from build123d import *

# Parameters (mm, degrees)
SKETCH1_W               = 95.2
SKETCH1_H               = 59.2
BOSS_EXTRUDE1_DEPTH     = 2
SKETCH2_R               = 6.5
CUT_EXTRUDE2_DEPTH      = 1
CUT_EXTRUDE2_DEPTH_BACK = 3
FILLET1_R               = 17.6


with BuildPart() as part:
    # Sketch1 → Boss-Extrude1 (new body)
    with BuildSketch(Plane(origin=(0, 0, 0), x_dir=(0, 1, 0), z_dir=(0, 0, 1))):
        with Locations((0, 29.6)):
            Rectangle(SKETCH1_W, SKETCH1_H)
    extrude(amount=BOSS_EXTRUDE1_DEPTH)

    # Sketch2 → Cut-Extrude2 (cut, two sides)
    with BuildSketch(Plane.XY.offset(2)) as cut_extrude2_sk:
        with Locations((-29.6, 0)):
            Circle(SKETCH2_R)
        with Locations((-46.6, 0)):
            Circle(SKETCH2_R)
        with Locations((-12.6, 0)):
            Circle(SKETCH2_R)
        with Locations((-12.6, -17)):
            Circle(SKETCH2_R)
        with Locations((-46.6, -17)):
            Circle(SKETCH2_R)
        with Locations((-29.6, -17)):
            Circle(SKETCH2_R)
        with Locations((-12.6, -34)):
            Circle(SKETCH2_R)
        with Locations((-46.6, -34)):
            Circle(SKETCH2_R)
        with Locations((-29.6, -34)):
            Circle(SKETCH2_R)
        with Locations((-46.6, 17)):
            Circle(SKETCH2_R)
        with Locations((-29.6, 17)):
            Circle(SKETCH2_R)
        with Locations((-12.6, 17)):
            Circle(SKETCH2_R)
        with Locations((-46.6, 34)):
            Circle(SKETCH2_R)
        with Locations((-29.6, 34)):
            Circle(SKETCH2_R)
        with Locations((-12.6, 34)):
            Circle(SKETCH2_R)
    extrude(amount=CUT_EXTRUDE2_DEPTH, mode=Mode.SUBTRACT)
    extrude(cut_extrude2_sk.sketch, amount=-CUT_EXTRUDE2_DEPTH_BACK, mode=Mode.SUBTRACT)

    # Fillet1
    fillet1_edges = [part.edges().sort_by_distance(p)[0] for p in [
        (-59.2, -47.6, 1),
        (-59.2, 47.6, 1),
        (0, 47.6, 1),
        (0, -47.6, 1),
    ]]
    fillet(fillet1_edges, radius=FILLET1_R)


solid = part.part
For this review, take the finished solid that the model builds, in its own axes (mm). Coordinates: 2 decimals unless noted, no trailing zeros. Loops run counter-clockwise (first coordinate to the right, second up) from the corner with the lowest first, then second, coordinate; pieces in that order, holes last. Notation, with made-up numbers: (72.25, 88.25) - (81.25, 88.25) arc R34 ccw to (81.25, 118.25) - close; hole circle Ø10 at (-27, 47). An arc over 180 degrees is marked (long way). Use a Markdown table: item, result. Add a question column.
Item 1: We need section D-D (y = -34). Give the boundary of the cut face in (x, z).
Item 2: We need section B-B (z = 1.15). Give the number of separate pieces and of enclosed holes in the cut face, and give its area (3 significant figures).
Item 3: We need section C-C (x = -34). Give the boundary of the cut face in (y, z).
Item 4: Mouldability with a two-part tool opening along X and no side actions: class faces 1 (the face through (-54.18, 42.31, 1.01)), 2 (the face through (-13.446, -27.555, 1.014)), 3 (the face through (-37, -1, 2)) as pulls with the +X half, pulls with the -X half, needs draft (parallel to the pull), parting line crosses it, or undercut.
Item 5: We need section A-A (y = 17). Give the boundary of the cut face in (x, z).
Item 6: Insertion check: pin 1 Ø8 at (x, y) = (-29.6, -17) entering from -Z. The pin has a flat end and moves straight along its axis. Give the tip position at first contact, or say it passes through.
Item 7: For line 1 (Y direction, x = -29.6, z = 0.6); line 2 (Y direction, x = -28, z = 1.45); line 3 (X direction, y = -0.5, z = 1.3), list the stretches that pass through material, from the lowest coordinate up.
Results list:
| question | item | result |
|---|---|---|
| 1 | outline | (-58.74, 0) - (-53.1, 0) - (-53.1, 2) - (-58.74, 2) - close; (-40.1, 0) - (-36.1, 0) - (-36.1, 2) - (-40.1, 2) - close; (-23.1, 0) - (-19.1, 0) - (-19.1, 2) - (-23.1, 2) - close; (-6.1, 0) - (-0.46, 0) - (-0.46, 2) - (-6.1, 2) - close |
| 2 | separate pieces | 1 |
| 2 | enclosed holes | 15 |
| 2 | area | 3,380 mm^2 |
| 3 | outline | (-47.6, 0) - (-38.78, 0) - (-38.78, 2) - (-47.6, 2) - close; (-29.22, 0) - (-21.78, 0) - (-21.78, 2) - (-29.22, 2) - close; (-12.22, 0) - (-4.78, 0) - (-4.78, 2) - (-12.22, 2) - close; (4.78, 0) - (12.22, 0) - (12.22, 2) - (4.78, 2) - close; (21.78, 0) - (29.22, 0) - (29.22, 2) - (21.78, 2) - close; (38.78, 0) - (47.6, 0) - (47.6, 2) - (38.78, 2) - close |
| 4 | face 1 | pulls with the -X half |
| 4 | face 2 | undercut |
| 4 | face 3 | needs draft |
| 5 | outline | (-59.2, 0) - (-53.1, 0) - (-53.1, 2) - (-59.2, 2) - close; (-40.1, 0) - (-36.1, 0) - (-36.1, 2) - (-40.1, 2) - close; (-23.1, 0) - (-19.1, 0) - (-19.1, 2) - (-23.1, 2) - close; (-6.1, 0) - (0, 0) - (0, 2) - (-6.1, 2) - close |
| 6 | pin 1 | passes through |
| 7 | line 1 | y = -47.6 to -40.5, -27.5 to -23.5, -10.5 to -6.5, 6.5 to 10.5, 23.5 to 27.5, 40.5 to 47.6 |
| 7 | line 2 | y = -47.6 to -40.3, -27.7 to -23.3, -10.7 to -6.3, 6.3 to 10.7, 23.3 to 27.7, 40.3 to 47.6 |
| 7 | line 3 | x = -59.2 to -53.08, -40.12 to -36.08, -23.12 to -19.08, -6.12 to 0 |
